Source: CAD feature listing. Evaluate the final solid. Frame: model axes, mm. A direction names the side the tool comes from. Round coordinates to 2 decimals unless told otherwise and drop trailing zeros. Write each loop counter-clockwise with the first axis right and the second up, starting at its lowest first coordinate (ties: lowest second). Pieces come first, ordered by that corner, then holes. Notation, with made-up numbers: (-38.75, 60) -> (-22.75, 60) arc R22 ccw to (-22.75, 72) -> close; hole circle Ø3 at (17.5, -10.5). An arc over 180 degrees is marked (long way). Return JSON: item names as keys, results as strings. Group by question number.
from build123d import *

# Parameters (mm, degrees)
SKETCH_9_R               = 30
EXTRUDE_3_DEPTH          = 15
EXTRUDE_4_DEPTH          = 12
FILLET_2_R               = 16
HOLE_WIZARD_M8_2_D       = 6.8
HOLE_WIZARD_M8_2_DEPTH   = 15
PATTERN_CIRCULAR_2_COUNT = 4


with BuildPart() as part:
    # 草图9 → 凸台-拉伸3 (new body)
    with BuildSketch(Plane(origin=(0, 0, 0), x_dir=(1, 0, 0), z_dir=(0, 1, 0))):
        with BuildLine():
            Line((70, 71.414284285), (70, -71.414284285))
            ThreePointArc((70, -71.414284285), (-100, 0), (70, 71.414284285))
        make_face()
        with Locations(Location((0, 0, 0), (0, 0, 270))):
            Circle(SKETCH_9_R, mode=Mode.SUBTRACT)
    extrude(amount=EXTRUDE_3_DEPTH)

    # 草图11 → 凸台-拉伸4 (add)
    with BuildSketch(Plane(origin=(-41.25, 23.815698604, 0), x_dir=(0, 0, 1), z_dir=(-0.8660254037844398, 0.499999999999998, 0))):
        with BuildLine():
            Line((-60, -9.97981973), (-60, 70.02018027))
            ThreePointArc((-60, 70.02018027), (-54.142135624, 84.162315894), (-40, 90.02018027))
            Line((-40, 90.02018027), (40, 90.02018027))
            ThreePointArc((40, 90.02018027), (54.142135624, 84.162315894), (60, 70.02018027))
            Line((60, 70.02018027), (60, -9.97981973))
            Line((60, -9.97981973), (52, -9.97981973))
            Line((52, -9.97981973), (52, 55.02018027))
            ThreePointArc((52, 55.02018027), (49.071067812, 62.091248082), (42, 65.02018027))
            Line((42, 65.02018027), (-42, 65.02018027))
            ThreePointArc((-42, 65.02018027), (-49.071067812, 62.091248082), (-52, 55.02018027))
            Line((-52, 55.02018027), (-52, -9.97981973))
            Line((-52, -9.97981973), (-60, -9.97981973))
        make_face()
    extrude(amount=-EXTRUDE_4_DEPTH)

    # 圆角2
    fillet_2_edges = [part.edges().sort_by_distance(p)[0] for p in [
        (-32.483339502, 15, -56),
        (-32.483339502, 15, 56),
    ]]
    fillet(fillet_2_edges, radius=FILLET_2_R)

    # M8 螺纹孔2
    with Locations(Plane(origin=(0, 15, 0), x_dir=(1, 0, 0), z_dir=(0, 1, 0))):
        with Locations((-60, 0)):
            hole_wizard_m8_2 = Hole(HOLE_WIZARD_M8_2_D / 2, depth=HOLE_WIZARD_M8_2_DEPTH)

    # 阵列(圆周)2: M8 螺纹孔2 ×4 about axis, 1 skipped
    pattern_circular_2_axis = Axis((0, 0, 0), (0, 1, 0))
    add([hole_wizard_m8_2.rotate(pattern_circular_2_axis, i * 360 / PATTERN_CIRCULAR_2_COUNT) for i in range(1, PATTERN_CIRCULAR_2_COUNT) if i not in (2,)], mode=Mode.SUBTRACT)


solid = part.part
Item 1: Set-up query: faces 4 (the cylindrical face through (-5.12, 74.56, 49.15)), 5 (the flat face through (-21, 47, 60)), 6 (the flat face through (5.276, 80.402, 0.84)). Return all of +Z, -Z, +X, -X, +Y, -Y with unobstructed straight access to the full face (end or side cutting, diameter ignored); none if empty.
Item 2: Cut plane D-D on y = 10. Output: boundary loops of the cut face in (x, z), and give its area (3 significant figures).
Item 3: Cut plane B-B on z = 0. Output: boundary loops of the cut face in (x, y).
Item 4: Pull-direction query (Z, two-part tool) for faces 1 (the flat face through (-22, 46, -60)), 2 (the cylindrical face through (1.3, 7.4, 63.14)), 3 (the cylindrical face through (-18.74, 23.2, -55.94)); classes: +Z half, -Z half, draft (parallel to the pull), parting line (faces both ways), or undercut.
Item 5: Material intervals for probe 1 along Y at (x, z) = (4.5, -84); probe 2 along X at (y, z) = (8.5, 57.5); probe 3 along X at (y, z) = (5, -60), sorted ascending.
Item 6: Cut plane A-A on x = -60. Output: boundary loops of the cut face in (y, z).
Item 7: Cut plane C-C on y = 22. Output: boundary loops of the cut face in (x, z), and give its area (3 significant figures).
Item 8: First-contact query: pin 1 Ø21.5 at (x, y) = (-26.5, 55) entering from -Z; pin 2 Ø6 at (y, z) = (47, 64.5) entering from -X; pin 3 Ø6 at (x, z) = (-39.5, -34.5) entering from +Y; pin 4 Ø4 at (y, z) = (74.5, -55.5) entering from -X. Flat tips, straight axial feed; report the tip coordinate or a pass-through.
Here are the results:
{
 "1": {"face 4": "-X", "face 5": "+Z, +X, -X, +Y", "face 6": "+Z, -Z, +X"},
 "2": {"outline": "(70, -71.41) -> (70, 71.41) arc R100 ccw (long way) to start; hole circle Ø6.8 at (-60, 0); hole circle Ø60 at (0, 0); hole circle Ø6.8 at (0, -60); hole circle Ø6.8 at (0, 60)", "area": "25,500 mm^2"},
 "3": {"outline": "(-100, 0) -> (-63.4, 0) -> (-63.4, 15) -> (-100, 15) -> close; (-56.6, 0) -> (-30, 0) -> (-30, 15) -> (-56.6, 15) -> close; (-8.74, 80.12) -> (1.65, 74.12) -> (14.15, 95.78) -> (3.76, 101.78) -> close; (30, 0) -> (70, 0) -> (70, 15) -> (30, 15) -> close"},
 "4": {"face 1": "-Z half", "face 2": "undercut", "face 3": "draft"},
 "5": {"probe 1": "y = 0 to 15", "probe 2": "x = -81.82 to -2.3, 2.3 to 70", "probe 3": "x = -80 to -3.4, 3.4 to 70"},
 "6": {"outline": "(0, -80) -> (15, -80) -> (15, -3.4) -> (0, -3.4) -> close; (0, 3.4) -> (15, 3.4) -> (15, 80) -> (0, 80) -> close"},
 "7": {"outline": "(-42.3, -60) -> (-18, -60) -> (-18, -52) -> (-42.3, -52) -> close; (-42.3, 52) -> (-18, 52) -> (-18, 60) -> (-42.3, 60) -> close", "area": "389 mm^2"},
 "8": {"pin 1": "stops at z = -60", "pin 2": "passes through", "pin 3": "stops at y = 15", "pin 4": "stops at x = -13.14"}
}
